Can you work these out from the model? Positions are in its coordinate system, mm. A direction names the side the tool comes from. Round coordinates to 2 decimals unless told otherwise and drop trailing zeros. Write each loop counter-clockwise with the first axis right and the second up, starting at its lowest first coordinate (ties: lowest second). Pieces come first, ordered by that corner, then holes. Notation, with made-up numbers: M 35.5,-29 L 61.5,-29 A27 cw 61.5,-9 Z; hole C 51,69.5 d8. An arc over 180 degrees is marked long. Answer in a Markdown table with one row per item. Add a question column.
(1) For faces 1 (the face through (-59, 2.5, -25)), 2 (the face through (-24, 8, -26.79)), 3 (the face through (-38.883, 7.632, -36.678)), 4 (the face through (-59, 12.5, -25)), 5 (the face through (-59, 8, -26.79)), which set-ups out of +Z, -Z, +X, -X, +Y, -Y let a thin tool reach every point of the face, with its end or its side?
(2) Suppose I cut it at D-D, the plane y = 13.5. Write out the boundary of the cut face in (x, z).
(3) If I drill on probe 1 along Z at (x, y) = (-55.5, 3.5); probe 2 along Z at (x, y) = (-57.5, 12.25); probe 3 along X at (y, z) = (12.5, -28.5), over which ranges is the centre line in solid material (lowest first)?
(4) I'm going to push flat-ended pins straight in: pin 1 (1.5 mm diameter, centred on x = -25, y = 10, fed in from -Z); pin 2 (2.5 mm diameter, centred on x = -32.88, y = 7.5, fed in from -Z); pin 3 (2 mm diameter, centred on x = -42, z = -31.5, fed in from -Y); pin 4 (8 mm diameter, centred on x = -31, z = -34, fed in from -Y). Where does each tip first touch, or does it pass through?
(5) Suppose I cut it at A-A, the plane y = 6. Write out the boundary of the cut face in (x, z).
(6) Suppose I cut it at C-C, the plane x = -40. Write out the boundary of the cut face in (y, z).
(7) If we mould it in two halves opening along Y, with no side actions, what happens to faces 6 (the face through (-24, 2.5, -25)), 7 (the face through (-21.881, 7, -25)), 8 (the face through (-47.143, 8.176, -26.325))? For each: released by +Y, released by -Y, zero draft, split by the parting line, or undercut.
(8) Suppose I cut it at B-B, the plane z = -37. Write out the boundary of the cut face in (x, y).
from build123d import *

# Parameters (mm, degrees)
SKETCH1_W           = 30
SKETCH1_H           = 5
BOSS_EXTRUDE1_DEPTH = 15
SKETCH3_R           = 1
CUT_EXTRUDE2_DEPTH  = 5
SKETCH5_W           = 5
SKETCH5_H           = 10
BOSS_EXTRUDE2_DEPTH = 3
SKETCH4_R           = 3
BOSS_EXTRUDE3_DEPTH = 16


with BuildPart() as part:
    # Sketch1 → Boss-Extrude1 (new body)
    with BuildSketch(Plane(origin=(0, 0, 0), x_dir=(1, 0, 0), z_dir=(0, 1, 0))):
        with Locations((-41.880536913, 26.290268456)):
            Rectangle(SKETCH1_W, SKETCH1_H)
    extrude(amount=BOSS_EXTRUDE1_DEPTH)

    # Sketch3 → Cut-Extrude2 (cut)
    with BuildSketch(Plane(origin=(0, 0, -28.790268456), x_dir=(-1, 0, 0), z_dir=(0, 0, -1))):
        with Locations((35.880536913, 7.5)):
            Circle(SKETCH3_R)
        with Locations((32.880536913, 7.5)):
            Circle(SKETCH3_R)
        with Locations((29.880536913, 7.5)):
            Circle(SKETCH3_R)
        with Locations((53.880536913, 7.5)):
            Circle(SKETCH3_R)
        with Locations((50.880536913, 7.5)):
            Circle(SKETCH3_R)
        with Locations((47.880536913, 7.5)):
            Circle(SKETCH3_R)
    extrude(amount=-CUT_EXTRUDE2_DEPTH, mode=Mode.SUBTRACT)

    # Sketch5 → Boss-Extrude2 (add)
    with BuildSketch(Plane.XY.offset(-23.790268456)):
        with Locations((-59.380536913, 7.5)):
            Rectangle(SKETCH5_W, SKETCH5_H)
        with Locations((-24.380536913, 7.5)):
            Rectangle(SKETCH5_W, SKETCH5_H)
    extrude(amount=-BOSS_EXTRUDE2_DEPTH)

    # Sketch4 → Boss-Extrude3 (add)
    with BuildSketch(Plane(origin=(0, 0, -28.790268456), x_dir=(-1, 0, 0), z_dir=(0, 0, -1))):
        with Locations((41.880536913, 7.5)):
            Circle(SKETCH4_R)
    extrude(amount=BOSS_EXTRUDE3_DEPTH)


solid = part.part
Calculated:
| question | item | result |
|---|---|---|
| 1 | face 1 | +Z, -Z, -X, -Y |
| 1 | face 2 | -Z, +X, +Y, -Y |
| 1 | face 3 | -Z |
| 1 | face 4 | +Z, -Z, -X, +Y |
| 1 | face 5 | -Z, -X, +Y, -Y |
| 2 | outline | M -56.88,-28.79 L -26.88,-28.79 L -26.88,-23.79 L -56.88,-23.79 Z |
| 3 | probe 1 | -28.79 to -23.79 |
| 3 | probe 2 | -26.79 to -23.79 |
| 3 | probe 3 | -56.88 to -26.88 |
| 4 | pin 1 | z = -26.79 |
| 4 | pin 2 | z = -28.79 |
| 4 | pin 3 | y = 4.5 |
| 4 | pin 4 | through |
| 5 | outline | M -61.88,-26.79 L -56.88,-26.79 L -56.88,-28.79 L -44.48,-28.79 L -44.48,-44.79 L -39.28,-44.79 L -39.28,-28.79 L -26.88,-28.79 L -26.88,-26.79 L -21.88,-26.79 L -21.88,-23.79 L -61.88,-23.79 Z |
| 6 | outline | M 0,-28.79 L 5.16,-28.79 L 5.16,-44.79 L 9.84,-44.79 L 9.84,-28.79 L 15,-28.79 L 15,-23.79 L 0,-23.79 Z |
| 7 | face 6 | released by -Y |
| 7 | face 7 | zero draft |
| 7 | face 8 | undercut |
| 8 | outline | C -41.88,7.5 d6 |
